```python
from build123d import *

# Parameters (mm, degrees)
SKETCH1_R           = 75
BOSS_EXTRUDE1_DEPTH = 10
SKETCH2_R           = 2.5
SKETCH2_R_2         = 3.75
BOSS_EXTRUDE2_DEPTH = 205
SKETCH3_R           = 75
BOSS_EXTRUDE3_DEPTH = 5
CUT_EXTRUDE1_REACH  = 246.233
SKETCH4_R           = 5


with BuildPart() as part:
    # Sketch1 → Boss-Extrude1 (new body)
    with BuildSketch(Plane(origin=(0, 0, 0), x_dir=(1, 0, 0), z_dir=(0, 1, 0))):
        with Locations(Location((0, 0, 0), (0, 0, 270))):
            Circle(SKETCH1_R)
    extrude(amount=BOSS_EXTRUDE1_DEPTH)

    # Sketch2 → Boss-Extrude2 (add)
    with BuildSketch(Plane(origin=(0, 10, 0), x_dir=(1, 0, 0), z_dir=(0, 1, 0))):
        with Locations(Location((-45.961940777, 45.961940777, 0), (0, 0, 90))):
            Circle(SKETCH2_R)
        with Locations(Location((45.961940777, 45.961940777, 0), (0, 0, 90))):
            Circle(SKETCH2_R)
        with Locations(Location((45.961940777, -45.961940777, 0), (0, 0, 90))):
            Circle(SKETCH2_R)
        with Locations(Location((-45.961940777, -45.961940777, 0), (0, 0, 90))):
            Circle(SKETCH2_R)
        with Locations(Location((38.961940777, 0, 0), (0, 0, 90))):
            Circle(SKETCH2_R_2)
    extrude(amount=BOSS_EXTRUDE2_DEPTH)

    # Sketch3 → Boss-Extrude3 (add)
    with BuildSketch(Plane(origin=(0, 215, 0), x_dir=(1, 0, 0), z_dir=(0, 1, 0))):
        with Locations(Location((0, 0, 0), (0, 0, 270))):
            Circle(SKETCH3_R)
    extrude(amount=BOSS_EXTRUDE3_DEPTH)

    # Sketch4 → Cut-Extrude1 (cut, up to next)
    with BuildSketch(Plane.XZ, mode=Mode.PRIVATE) as cut_extrude1_sk1:
        with Locations(Location((0, 0, 0), (0, 0, 270))):
            Circle(SKETCH4_R)
    cut_extrude1_tool1 = extrude(cut_extrude1_sk1.sketch, amount=-CUT_EXTRUDE1_REACH, mode=Mode.PRIVATE) & part.part
    add(cut_extrude1_tool1.solids().sort_by_distance((0, 0, 0))[0], mode=Mode.SUBTRACT)


solid = part.part
```
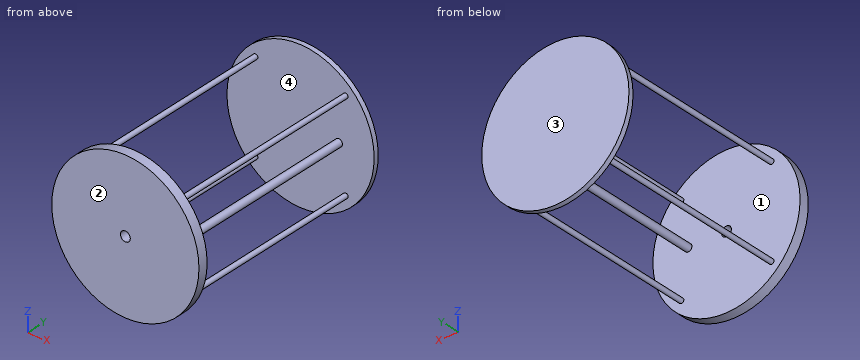
Can you work these out from the model? Positions are in its coordinate system, mm. Face numbers are marked on the shaded views. Coordinates: 2 decimals unless noted, no trailing zeros. Loops run counter-clockwise (first coordinate to the right, second up) from the corner with the lowest first, then second, coordinate; pieces in that order, holes last.
1) I need wall thicknesses on probe 1 along Y at (x, z) = (23.5, 51); probe 2 along X at (y, z) = (7, 0); probe 3 along X at (y, z) = (56.5, -48). Which ranges of each line are inside material? Lowest first, please.
2) Imagine slicing it at B-B on z = 0. List the corners of the cut face in (x, y) for me.
3) Imagine slicing it at D-D on x = -18. List the corners of the cut face in (y, z) for me, plus the area to 3 significant figures.
4) Imagine slicing it at C-C on y = 122. List the corners of the cut face in (x, z) for me.
5) Imagine slicing it at A-A on x = 0. List the corners of the cut face in (y, z) for me.
6) For pin 1 (12 mm diameter, centred on y = 95, z = 32.5, fed in from +X), with a flat end and sliding along its axis, tell me the tip position at first contact or that it passes through.
7) Thinking about a two-plate mould opening in Y: for the marked faces 1, 2, 3 and 4, which applies, pulls with the +Y half, pulls with the -Y half, needs draft (parallel to the pull), parting line crosses it, or undercut?
Completed:
1. probe 1: y = 0 to 10, 215 to 220
1. probe 2: x = -75 to -5, 5 to 75
1. probe 3: x = -47.41 to -44.51, 44.51 to 47.41
2. outline: (-75, 0) - (-5, 0) - (-5, 10) - (-75, 10) - close; (-75, 215) - (35.21, 215) - (35.21, 10) - (5, 10) - (5, 0) - (75, 0) - (75, 10) - (42.71, 10) - (42.71, 215) - (75, 215) - (75, 220) - (-75, 220) - close
3. outline: (0, -72.81) - (10, -72.81) - (10, 72.81) - (0, 72.81) - close; (215, -72.81) - (220, -72.81) - (220, 72.81) - (215, 72.81) - close
3. area: 2,180 mm2
4. outline: circle Ø5 at (-45.96, -45.96); circle Ø5 at (-45.96, 45.96); circle Ø7.5 at (38.96, 0); circle Ø5 at (45.96, -45.96); circle Ø5 at (45.96, 45.96)
5. outline: (0, -75) - (10, -75) - (10, -5) - (0, -5) - close; (0, 5) - (10, 5) - (10, 75) - (0, 75) - close; (215, -75) - (220, -75) - (220, 75) - (215, 75) - close
6. pin 1: passes through
7. face 1: undercut
7. face 2: pulls with the -Y half
7. face 3: pulls with the +Y half
7. face 4: undercut
